from build123d import *

# Parameters (mm, degrees)
BOSS_EXTRUDE1_DEPTH = 71.12
SKETCH2_R           = 6
CUT_EXTRUDE1_DEPTH  = 4
CUT_EXTRUDE2_REACH  = 76.031
SKETCH3_R           = 2.16
CUT_EXTRUDE3_REACH  = 76.436
SKETCH5_W           = 7.8486
SKETCH5_H           = 7.8486


with BuildPart() as part:
    # Sketch1 → Boss-Extrude1 (new body)
    with BuildSketch(Plane.XY):
        Polygon((9.127895876, 7.8486), (9.127895876, 0), (12.556895876, 0), (12.556895876, -11.9507), (18.652895876, -11.9507), (18.652895876, 19.7993), (12.556895876, 19.7993), (12.556895876, 7.8486), align=None)
    extrude(amount=BOSS_EXTRUDE1_DEPTH)

    # Sketch2 → Cut-Extrude1 (cut)
    with BuildSketch(Plane.ZY.offset(-9.127895876)):
        with Locations((16.51, 3.9243)):
            Circle(SKETCH2_R)
        with Locations((54.61, 3.9243)):
            Circle(SKETCH2_R)
    extrude(amount=-CUT_EXTRUDE1_DEPTH, mode=Mode.SUBTRACT)

    # Sketch3 → Cut-Extrude2 (cut, up to next)
    with BuildSketch(Plane.ZY.offset(-13.127895876), mode=Mode.PRIVATE) as cut_extrude2_sk1:
        with Locations((16.51, 3.9243)):
            Circle(SKETCH3_R)
    cut_extrude2_tool1 = extrude(cut_extrude2_sk1.sketch, amount=-CUT_EXTRUDE2_REACH, mode=Mode.PRIVATE) & part.part
    # Sketch3 → Cut-Extrude2 (cut, up to next)
    with BuildSketch(Plane.ZY.offset(-13.127895876), mode=Mode.PRIVATE) as cut_extrude2_sk2:
        with Locations((54.61, 3.9243)):
            Circle(SKETCH3_R)
    cut_extrude2_tool2 = extrude(cut_extrude2_sk2.sketch, amount=-CUT_EXTRUDE2_REACH, mode=Mode.PRIVATE) & part.part
    add(cut_extrude2_tool1.solids().sort_by_distance((13.127896, 3.9243, 16.51))[0], mode=Mode.SUBTRACT)
    add(cut_extrude2_tool2.solids().sort_by_distance((13.127896, 3.9243, 54.61))[0], mode=Mode.SUBTRACT)

    # Sketch5 → Cut-Extrude3 (cut, up to next)
    with BuildSketch(Plane.ZY.offset(-9.127895876), mode=Mode.PRIVATE) as cut_extrude3_sk1:
        with Locations((35.56, 3.9243)):
            Rectangle(SKETCH5_W, SKETCH5_H)
    cut_extrude3_tool1 = extrude(cut_extrude3_sk1.sketch, amount=-CUT_EXTRUDE3_REACH, mode=Mode.PRIVATE) & part.part
    add(cut_extrude3_tool1.solids().sort_by_distance((9.127896, 3.9243, 35.56))[0], mode=Mode.SUBTRACT)


solid = part.part
Can you work these out from the model? Positions are in its coordinate system, mm. A direction names the side the tool comes from. Round coordinates to 2 decimals unless told otherwise and drop trailing zeros. Write each loop counter-clockwise with the first axis right and the second up, starting at its lowest first coordinate (ties: lowest second). Pieces come first, ordered by that corner, then holes. Notation, with made-up numbers: (-36, -8.5) -> (-26, -8.5) arc R14 ccw to (-26, 18.5) -> close; hole circle Ø3 at (55, 21). An arc over 180 degrees is marked (long way). Use one line per item in the form item = value. Start each with the question number.
Q1. Imagine slicing it at C-C (y = 5). Please give me the cut outline in (x, z).
Q2. Imagine slicing it at A-A (x = 10). Please give me the cut outline in (y, z).
Q3. If I drill on probe 1 along Y at (x, z) = (16.5, 54.61); probe 2 along Z at (x, y) = (12.5, 2); probe 3 along Z at (x, y) = (10.75, 4.5), over which ranges is the centre line in solid material (lowest first)? Write a range as [from, to].
Q4. Imagine slicing it at D-D (x = 15.25). Please give me the cut outline in (y, z), then the cut area to 3 significant figures.
Q5. Imagine slicing it at B-B (z = 16.51). Please give me the cut outline in (x, y).
Q6. We'd pull the mould along Z, two halves only. Please class faces 1 (the face through (11, 7.849, 6)), 2 (the face through (15, 4, 0)), 3 (the face through (15.852, 4.019, 52.452)): +Z half, -Z half, draft (parallel to the pull), parting line (faces both ways), or undercut.
Q7. Which directions (+Z, -Z, +X, -X, +Y, -Y) give clear straight access to the entire face, cutting with the end or side of a thin tool? Please do faces 4 (the face through (13.128, 4, 19)), 5 (the face through (11, 0, 65)), 6 (the face through (14, 4, 31.636)), 7 (the face through (11, 7.849, 65)).
Q8. I'm going to push flat-ended pins straight in: P1, Ø1, axis at x = 10.5, z = 47, coming from the +Y side; P2, Ø3.5, axis at y = 3.92, z = 54.61, coming from the +X side; P3, Ø11, axis at y = 3.92, z = 16.51, coming from the -X side; P4, Ø1, axis at x = 11.5, z = 45, coming from the -Y side. Where does each tip first touch, or does it pass through?
Worked out:
q1.outline = (9.13, 0) -> (18.65, 0) -> (18.65, 14.64) -> (13.13, 14.64) -> (13.13, 10.61) -> (9.13, 10.61) -> close; (9.13, 22.41) -> (13.13, 22.41) -> (13.13, 18.38) -> (18.65, 18.38) -> (18.65, 31.64) -> (9.13, 31.64) -> close; (9.13, 39.48) -> (18.65, 39.48) -> (18.65, 52.74) -> (13.13, 52.74) -> (13.13, 48.71) -> (9.13, 48.71) -> close; (9.13, 60.51) -> (13.13, 60.51) -> (13.13, 56.48) -> (18.65, 56.48) -> (18.65, 71.12) -> (9.13, 71.12) -> close
q2.outline = (0, 0) -> (7.85, 0) -> (7.85, 11.97) arc R6 cw to (0, 11.97) -> close; (0, 21.05) arc R6 cw to (7.85, 21.05) -> (7.85, 31.64) -> (0, 31.64) -> close; (0, 39.48) -> (7.85, 39.48) -> (7.85, 50.07) arc R6 cw to (0, 50.07) -> close; (0, 59.15) arc R6 cw to (7.85, 59.15) -> (7.85, 71.12) -> (0, 71.12) -> close
q3.probe_1 = [-11.95, 1.76], [6.08, 19.8]
q3.probe_2 = [0, 10.83], [22.19, 31.64], [39.48, 48.93], [60.29, 71.12]
q3.probe_3 = [0, 10.54], [22.48, 31.64], [39.48, 48.64], [60.58, 71.12]
q4.outline = (-11.95, 0) -> (19.8, 0) -> (19.8, 71.12) -> (-11.95, 71.12) -> close; hole (0, 31.64) -> (7.85, 31.64) -> (7.85, 39.48) -> (0, 39.48) -> close; hole circle Ø4.32 at (3.92, 16.51); hole circle Ø4.32 at (3.92, 54.61)
q4.area = 2,170 mm^2
q5.outline = (12.56, -11.95) -> (18.65, -11.95) -> (18.65, 1.76) -> (13.13, 1.76) -> (13.13, -2.08) -> (12.56, -2.08) -> close; (12.56, 9.92) -> (13.13, 9.92) -> (13.13, 6.08) -> (18.65, 6.08) -> (18.65, 19.8) -> (12.56, 19.8) -> close
q6.face_1 = draft
q6.face_2 = -Z half
q6.face_3 = undercut
q7.face_4 = -X
q7.face_5 = +Z, -Z, -X, -Y
q7.face_6 = +X, -X
q7.face_7 = +Z, -Z, -X, +Y
q8.P1 = 7.85
q8.P2 = through
q8.P3 = 13.13
q8.P4 = 0
